from build123d import *

# Parameters (mm, degrees)
SKETCH1_R           = 5
BOSS_EXTRUDE1_DEPTH = 3
SKETCH2_W           = 22
SKETCH2_H           = 10
BOSS_EXTRUDE2_DEPTH = 3
SKETCH3_R           = 5
BOSS_EXTRUDE3_DEPTH = 3
BOSS_EXTRUDE4_DEPTH = 3
BOSS_EXTRUDE5_DEPTH = 3


with BuildPart() as part:
    # Sketch1 → Boss-Extrude1 (new body)
    with BuildSketch(Plane.XY):
        Circle(SKETCH1_R)
    extrude(amount=BOSS_EXTRUDE1_DEPTH)

    # Sketch2 → Boss-Extrude2 (add)
    with BuildSketch(Plane.XY):
        with Locations((11, 0)):
            Rectangle(SKETCH2_W, SKETCH2_H)
    extrude(amount=BOSS_EXTRUDE2_DEPTH)

    # Sketch3 → Boss-Extrude3 (add)
    with BuildSketch(Plane.XY):
        with Locations((22, 0)):
            Circle(SKETCH3_R)
    extrude(amount=BOSS_EXTRUDE3_DEPTH)

    # Sketch4 → Boss-Extrude4 (add)
    with BuildSketch(Plane.XY):
        Polygon((20.943454346, 2.265769468), (53.570534679, 17.48002689), (55.683625988, 12.948487955), (23.056545654, -2.265769468), align=None)
    extrude(amount=BOSS_EXTRUDE4_DEPTH)

    # Sketch5 → Boss-Extrude5 (add)
    with BuildSketch(Plane.XY):
        Polygon((54.627080333, 15.214257423), (69.128004926, 21.976149611), (74.199424067, 11.100456166), (59.698499474, 4.338563978), align=None)
    extrude(amount=BOSS_EXTRUDE5_DEPTH)


solid = part.part
Build history of the part. All positions in model axes, mm. A direction names the side the tool comes from. Coordinates: 2 decimals unless noted, no trailing zeros. Order: outer loops, then holes, each group sorted by start corner. A loop starts at its lowest first (then second) coordinate and runs counter-clockwise, first axis right, second up. Notation, with made-up numbers: (13.25, -11) - (38.25, -11) arc R11 ccw to (38.25, 10) - close; hole circle Ø6 at (54.25, 6). An arc over 180 degrees is marked (long way). Write item = value, one per line. Start each with the question number.
1) Saw through at C-C on x = 16.5. Write the cut outline in (y, z).
2) Wall check: line 1 along X through (y, z) = (17.25, 0.8); line 2 along X through (y, z) = (11.25, 2.4); line 3 along Y through (x, z) = (1, 1.75). Give the ranges that are in metal, low to high. Write a range as from..to.
3) Two-plate mould, pull along X, no slides. Class faces 5 (the face through (11, -5, 1)), 6 (the face through (67.05, 7.767, 1.479)), 7 (the face through (61.78, 18.55, 1.48)), 8 (the face through (57.72, 8.58, 1.48)): pulls with the +X half, pulls with the -X half, needs draft (parallel to the pull), parting line crosses it, or undercut.
4) Saw through at D-D on y = 5.75. Write the cut outline in (x, z).
5) Saw through at A-A on y = 9. Write the cut outline in (x, z), then the cut area to 3 significant figures.
6) 3-axis set-ups, long thin cutter, end or side, ignore diameter. For faces 1 (the face through (41.53, 6.35, 1.48)), 2 (the face through (35, 6, 0)), 3 (the face through (11, 5, 1)), 4 (the face through (23.524, 4.762, 1.479)): which of +Z, -Z, +X, -X, +Y, -Y reach the whole face in a straight line?
7) Saw through at B-B on z = 2.5. Write the cut outline in (x, y), then the cut area to 3 significant figures.
8) Flat gauge pins, fed straight in: pin 1 Ø1 at (x, z) = (26.5, 1) entering from +Y; pin 2 Ø0.9 at (x, z) = (16, 2) entering from +Y. Where does each tip first touch, or does it go through?
From the geometry:
q1.outline = (-5, 0) - (5, 0) - (5, 3) - (-5, 3) - close
q2.line_1 = 53.08..53.68, 58.99..71.33
q2.line_2 = 40.21..52.04, 56.48..74.13
q2.line_3 = -5..5
q3.face_5 = needs draft
q3.face_6 = pulls with the +X half
q3.face_7 = undercut
q3.face_8 = undercut
q4.outline = (28.42, 0) - (40.25, 0) - (40.25, 3) - (28.42, 3) - close; (59.04, 0) - (62.73, 0) - (62.73, 3) - (59.04, 3) - close
q5.outline = (35.39, 0) - (47.22, 0) - (47.22, 3) - (35.39, 3) - close; (57.52, 0) - (69.69, 0) - (69.69, 3) - (57.52, 3) - close
q5.area = 72.0 mm^2
q6.face_1 = +Z, -Z, -Y
q6.face_2 = -Z, +X, -X, +Y, -Y
q6.face_3 = +Z, -Z, -X, +Y
q6.face_4 = +Z, -Z, +Y
q7.outline = (0, -5) - (22, -5) arc R5 ccw to (26.98, -0.44) - (55.68, 12.95) - (59.7, 4.34) - (74.2, 11.1) - (69.13, 21.98) - (54.63, 15.21) - (53.57, 17.48) - (24.87, 4.1) arc R5 ccw to (22, 5) - (0, 5) arc R5 ccw to start
q7.area = 647 mm^2
q8.pin_1 = 5.09
q8.pin_2 = 5
